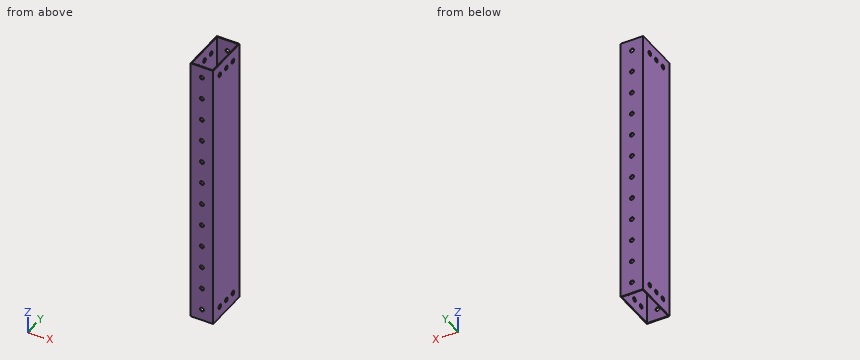
Autodesk Inventor part; units mm, degrees
ref_plane "YZ Plane" through (0, 0, 0) normal (1, 0, 0) x (0, 1, 0)
ref_plane "XZ Plane" through (0, 0, 0) normal (0, 1, 0) x (-1, 0, 0)
ref_plane "XY Plane" through (0, 0, 0) normal (0, 0, 1) x (1, 0, 0)
sketch "Sketch1" plane through (0, 0, 0) normal (0, 0, 1) x (1, 0, 0)
  line L0 (12.7, 25.4) -> (-12.7, 25.4)
  line L1 (-12.7, 25.4) -> (-12.7, -25.4)
  line L2 (-12.7, -25.4) -> (12.7, -25.4)
  line L3 (12.7, -25.4) -> (12.7, 25.4)
  line L4 (12.7, 25.4) -> (-12.7, -25.4) construction
  line L5 (-12.7, 25.4) -> (12.7, -25.4) construction
  line L6 (-11.684, 24.384) -> (11.684, 24.384)
  line L7 (11.684, 24.384) -> (11.684, -24.384)
  line L8 (11.684, -24.384) -> (-11.684, -24.384)
  line L9 (-11.684, -24.384) -> (-11.684, 24.384)
  point P0 (0, 0)
  dimension "d0" = 1.016
  dimension "d1" = 50.8
  dimension "d2" = 25.4
extrude "Tube Length" add sketch "Sketch1" along normal mid plane 304.8
sketch "Sketch2" plane through (-12.7, 25.4, 152.4) normal (0, 1, 0) x (1, 0, 0)
  line L0 (0, 0) -> (0, 304.8)
  line L1 (25.4, 0) -> (0, 0)
  line L2 (25.4, 304.8) -> (25.4, 0)
  line L3 (0, 304.8) -> (25.4, 304.8)
  line L4 (25.4, 0) -> (0, 0)
  line L5 (12.7, 0) -> (12.7, 12.7) construction
  circle A0 centre (12.7, 12.7) radius 2.2479
  point P0 (12.7, 152.4)
  dimension "d5" = 12.7
  dimension "d6" = 4.4958
extrude "Top Hole" cut sketch "Sketch2" against normal through all contours A0
pattern_linear "Rectangular Pattern1" count 12 spacing 25.4 along (0, 0, -1) of "Top Hole"
sketch "Sketch4" plane through (-12.7, -25.4, 152.4) normal (-1, 0, 0) x (0, 0, 1)
  line L0 (-304.8, 0) -> (0, 0)
  line L1 (0, 50.8) -> (0, 0)
  line L2 (0, 50.8) -> (-304.8, 50.8)
  line L3 (-304.8, 0) -> (-304.8, 50.8)
  line L4 (-304.8, 25.4) -> (-292.1, 25.4)
  line L5 (-152.4, 25.4) -> (-152.4, 13.4487)
  point P0 (-292.1, 12.7)
  point P1 (-292.1, 38.1)
  point P2 (-12.7, 12.7)
  point P3 (-12.7, 25.4)
  point P4 (-12.7, 38.1)
  dimension "d31" = 12.7
  dimension "d34" = 12.7
hole "Hole1" at (-12.7, -12.7, -139.7) at (-12.7, 0, -139.7) at (-12.7, 12.7, -139.7) at (-12.7, 12.7, 139.7) at (-12.7, -12.7, 139.7) at (-12.7, 0, 139.7) direction (1, 0, 0) diameter 5.1054 end through all
sketch "Sketch3" plane through (0, 0, 152.4) normal (0, 0, 1) x (1, 0, 0)
  line L0 (0, 0) -> (0, 25.4) construction
  line L1 (12.7, 25.4) -> (-12.7, 25.4)
  line L2 (-0.0508, 25.4) -> (0, 25.2984)
  line L3 (0.0508, 25.4) -> (0, 25.2984)
  line L4 (-12.7, 12.6492) -> (-12.5984, 12.7)
  line L5 (-12.7, 12.7508) -> (-12.5984, 12.7)
  line L6 (-12.7, -0.0508) -> (-12.5984, 0)
  line L7 (-12.7, 0.0508) -> (-12.5984, 0)
  line L8 (-12.7, -12.7508) -> (-12.5984, -12.7)
  line L9 (-12.7, -12.6492) -> (-12.5984, -12.7)
  line L10 (12.7, 0.0508) -> (12.5984, 0)
  line L11 (12.7, 12.6492) -> (12.5984, 12.7)
  line L12 (12.7, 12.7508) -> (12.5984, 12.7)
  line L13 (12.7, -0.0508) -> (12.5984, 0)
  line L14 (12.7, -12.6492) -> (12.5984, -12.7)
  line L15 (12.7, -12.7508) -> (12.5984, -12.7)
  line L16 (0.0508, -25.4) -> (0, -25.2984)
  line L17 (-0.0508, -25.4) -> (0, -25.2984)
  line L18 (-12.7, 25.4) -> (-12.7, -25.4)
  line L19 (12.7, -25.4) -> (12.7, 25.4)
  line L20 (-12.7, -25.4) -> (12.7, -25.4)
  point P0 (0, 12.7)
  point P1 (-12.7, 12.7)
  point P2 (-12.7, 0)
  point P3 (-12.7, -12.7)
  point P4 (12.7, 12.7)
  point P5 (12.7, 0)
  point P6 (12.7, -12.7)
  point P7 (0, -25.4)
  dimension "d12" = 0.1016
  dimension "d13" = 0.1016
  dimension "d16" = 90
  dimension "d20" = 12.7
  dimension "d27" = 360
equation "\"d13\" = d12"
properties part number "Elevator Stage 1 Gearbox Mounting Tube" material "Aluminum 6061"
Could you check a few things on this model? Use its own coordinates, in mm. Give positions to 0.01 mm unless a question says otherwise; leave off trailing zeros. Order: outer loops, then holes, each group sorted by start corner. A loop starts at its lowest first (then second) coordinate and runs counter-clockwise, first axis right, second up.
Item 1: I need wall thicknesses on line 1 (Y direction, x = 12, z = 139.7); line 2 (Y direction, x = 4.5, z = 110); line 3 (X direction, y = -22, z = 112.5). Which ranges of each line are inside material? Lowest first, please.
Item 2: If we section it at C-C, the plane z = 30: Write out the boundary of the cut face in (x, y).
Item 3: If we section it at B-B, the plane y = 7: Write out the boundary of the cut face in (x, z).
Item 4: If we section it at A-A, the plane x = 6.25: Write out the boundary of the cut face in (y, z).
Values:
1. line 1: y = -25.4 to -15.25, -10.15 to -2.55, 2.55 to 10.15, 15.25 to 25.4
1. line 2: y = -25.4 to -24.38, 24.38 to 25.4
1. line 3: x = -12.7 to -11.68, 11.68 to 12.7
2. outline: (-12.7, -25.4) - (12.7, -25.4) - (12.7, 25.4) - (-12.7, 25.4) - close; hole (-11.68, -24.38) - (11.68, -24.38) - (11.68, 24.38) - (-11.68, 24.38) - close
3. outline: (-12.7, -152.4) - (-11.68, -152.4) - (-11.68, 152.4) - (-12.7, 152.4) - close; (11.68, -152.4) - (12.7, -152.4) - (12.7, 152.4) - (11.68, 152.4) - close
4. outline: (-25.4, -152.4) - (-24.38, -152.4) - (-24.38, 152.4) - (-25.4, 152.4) - close; (24.38, -152.4) - (25.4, -152.4) - (25.4, 152.4) - (24.38, 152.4) - close
